Source: CAD feature listing. Evaluate the final solid. Frame: model axes, mm. Face numbers are marked on the shaded views. A direction names the side the tool comes from. Round coordinates to 2 decimals unless told otherwise and drop trailing zeros. Loops run counter-clockwise (first coordinate to the right, second up) from the corner with the lowest first, then second, coordinate; pieces in that order, holes last. Notation, with made-up numbers: M -33.5,63.25 L 13.5,63.25 A3 cw 13.5,67.25 Z; hole C 11,54.5 d1. An arc over 180 degrees is marked long. One line per item, written item: value.
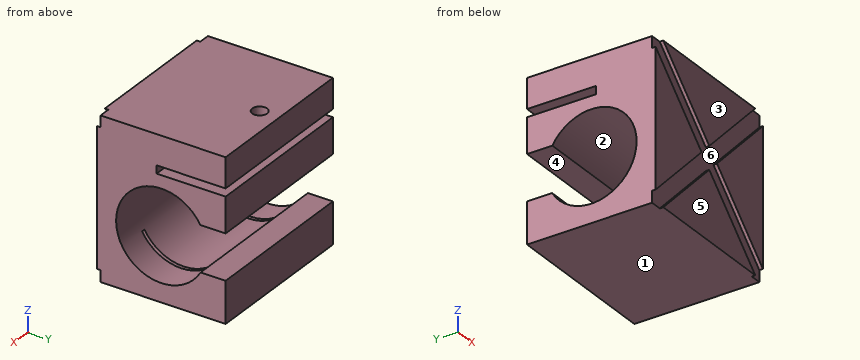
from build123d import *

# Parameters (mm, degrees)
F0_W          = 1701.8
F0_H          = 1701.8
F1_DEPTH      = 685.8
F1_DEPTH_BACK = 685.8
F3_R          = 482.6
F5_DEPTH      = 1778
F4_W          = 741.2019371986
F4_H          = 241.3
F6_DEPTH      = 1778
F7_W          = 762
F7_H          = 83.82
F8_DEPTH      = 1778
F10_DEPTH     = 38.1
F12_R         = 80.01
F13_DEPTH     = 320.04
F15_W         = 38.1
F15_H         = 1016
F16_DEPTH     = 304.8


with BuildPart() as f1:
    # F0 (on Front) → F1 (new body, two sides)
    with BuildSketch(Plane.XZ) as f1_sk:
        Rectangle(F0_W, F0_H)
    extrude(amount=F1_DEPTH)
    extrude(f1_sk.sketch, amount=-F1_DEPTH_BACK)

    # F3 (on face) → F5 (cut)
    with BuildSketch(Plane.YZ.offset(850.9)):
        with Locations((0, -170.704353589)):
            Circle(F3_R)
    extrude(amount=-F5_DEPTH, mode=Mode.SUBTRACT)

    # F4 (on face) → F6 (cut)
    with BuildSketch(Plane.YZ.offset(850.9)):
        with Locations((370.6009685993, -47.7492743492)):
            Rectangle(F4_W, F4_H)
        Polygon((741.2019371986, -168.3992743492), (0, -168.3992743492), (0, -409.6992743492), (741.8479657151, -409.6992743492), (741.8479657151, -168.3992743492), align=None)
    extrude(amount=-F6_DEPTH, mode=Mode.SUBTRACT)

    # F7 (on face) → F8 (cut)
    with BuildSketch(Plane.YZ.offset(850.9)):
        with Locations((330.9977193773, 490.6306193733)):
            Rectangle(F7_W, F7_H)
    extrude(amount=-F8_DEPTH, mode=Mode.SUBTRACT)

    # F9 (on face) → F10 (cut)
    with BuildSketch(Plane.XZ.offset(685.8)):
        Polygon((850.9, 728.98), (850.9, 850.9), (728.98, 850.9), (0, 121.92), (121.92, 0), align=None)
        Polygon((850.9, -728.98), (121.92, 0), (0, -121.92), (728.98, -850.9), (850.9, -850.9), align=None)
        Polygon((0, -121.92), (121.92, 0), (0, 121.92), (-121.92, 0), align=None)
        Polygon((-121.92, 0), (0, 121.92), (-728.98, 850.9), (-850.9, 850.9), (-850.9, 728.98), align=None)
        Polygon((-728.98, -850.9), (0, -121.92), (-121.92, 0), (-850.9, -728.98), (-850.9, -850.9), align=None)
    extrude(amount=-F10_DEPTH, mode=Mode.SUBTRACT)

    # F12 (on face) → F13 (cut)
    with BuildSketch(Plane.XY.offset(850.9)):
        with Locations((0, 476.8736362457)):
            Circle(F12_R)
    extrude(amount=-F13_DEPTH, mode=Mode.SUBTRACT)

    # F15 (on face) → F16 (cut)
    with BuildSketch(Plane.XY.offset(-409.6992743492)):
        with Locations((514.6490952492, -87.3333351612)):
            Rectangle(F15_W, F15_H)
        with Locations((-552.4504163742, -88.7147324085)):
            Rectangle(F15_W, F15_H)
    extrude(amount=-F16_DEPTH, mode=Mode.SUBTRACT)


solid = f1.part
1. Section query B-B (z = 205.5). Return the cut outline in (x, y), and give its area (3 significant figures).
Report:
outline: M -850.9,-685.8 L -327.42,-685.8 L -327.42,-647.7 L -83.58,-647.7 L -83.58,-685.8 L 83.58,-685.8 L 83.58,-647.7 L 327.42,-647.7 L 327.42,-685.8 L 850.9,-685.8 L 850.9,-302.28 L -850.9,-302.28 Z; M -850.9,302.28 L 850.9,302.28 L 850.9,685.8 L -850.9,685.8 Z
area: 1,290,000 mm2
2. Ray query, line 1 (Z direction, x = 488.5, y = 464.5); line 2 (X direction, y = 130, z = -645); line 3 (Z direction, x = 426, y = 0). Return the intervals inside material, ascending. Write a range as [from, to].
Report:
line 1: z = [-850.9, -409.7], [72.9, 448.72], [532.54, 850.9]
line 2: x = [-850.9, -571.5], [-533.4, 495.6], [533.7, 850.9]
line 3: z = [-850.9, -653.3], [311.9, 448.72], [532.54, 850.9]
3. Section query A-A (y = 65). Return the cut outline in (x, z), and give its area (3 significant figures).
Report:
outline: M -850.9,-850.9 L 850.9,-850.9 L 850.9,-648.91 L 533.7,-648.91 L 533.7,-714.5 L 495.6,-714.5 L 495.6,-648.91 L -533.4,-648.91 L -533.4,-714.5 L -571.5,-714.5 L -571.5,-648.91 L -850.9,-648.91 Z; M -850.9,307.5 L 850.9,307.5 L 850.9,448.72 L -850.9,448.72 Z; M -850.9,532.54 L 850.9,532.54 L 850.9,850.9 L -850.9,850.9 Z
area: 1,120,000 mm2
4. Section query D-D (x = -350). Return the cut outline in (y, z), and give its area (3 significant figures).
Report:
outline: M -685.8,-850.9 L 685.8,-850.9 L 685.8,-409.7 L 419.27,-409.7 A482.6 cw long 416.6,72.9 L 685.8,72.9 L 685.8,448.72 L -50,448.72 L -50,532.54 L 685.8,532.54 L 685.8,850.9 L -685.8,850.9 L -685.8,471.92 L -647.7,471.92 L -647.7,228.08 L -685.8,228.08 L -685.8,-228.08 L -647.7,-228.08 L -647.7,-471.92 L -685.8,-471.92 Z
area: 1,410,000 mm2
5. Pin query (flat end, axial travel): pin 1 (1.5 mm diameter, centred on x = 275, z = -384.5, fed in from -Y); pin 2 (8 mm diameter, centred on x = 86.5, z = -23.5, fed in from +Y). Return the tip coordinate at first contact, or that it passes through.
Report:
pin 1: stops at y = -647.7
pin 2: stops at y = -458.3
6. Pull-direction query (Z, two-part tool) for the marked faces 1, 2 and 3; classes: released by +Z, released by -Z, zero draft, split by the parting line, or undercut.
Report:
face 1: released by -Z
face 2: undercut
face 3: zero draft
7. Reachability of the marked faces 4, 5 and 6 from +Z, -Z, +X, -X, +Y, -Y: full face, straight path, thin tool, end or side. Return the list, or none.
Report:
face 4: +X, -X, +Y
face 5: +Z, -Z, +X, -X, -Y
face 6: -Y
8. Section query C-C (y = -305). Return the cut outline in (x, z).
Report:
outline: M -850.9,-850.9 L 850.9,-850.9 L 850.9,-544.71 L 533.7,-544.71 L 533.7,-714.5 L 495.6,-714.5 L 495.6,-544.71 L -533.4,-544.71 L -533.4,-714.5 L -571.5,-714.5 L -571.5,-544.71 L -850.9,-544.71 Z; M -850.9,203.3 L 850.9,203.3 L 850.9,850.9 L -850.9,850.9 Z
